from build123d import *

# Parameters (mm, degrees)
EXTRUDE_1_DEPTH        = 25
SKETCH_4_R             = 22
CUT_EXTRUDE_1_DEPTH    = 1.8
CUT_EXTRUDE_START      = 6
CUT_EXTRUDE_1_2_DEPTH  = 3
SKETCH_11_W            = 18.9
SKETCH_11_H            = 1.4
EXTRUDE_3_DEPTH        = 1.5
FILLET_1_R             = 0.25
SKETCH_12_R            = 1
CUT_EXTRUDE_2623_DEPTH = 91.722501261
CUT_EXTRUDE_1_3_DEPTH  = 1
SKETCH_14_W            = 0.8
SKETCH_14_H            = 6.2
CUT_EXTRUDE_2_DEPTH    = 1


with BuildPart() as part:
    # 草图2 → 整体拉伸-薄壁1 (new, symmetric)
    with BuildSketch(Plane.XY):
        with BuildLine():
            ThreePointArc((28.874192719, 5.049687275), (37.065713162, 9.313922912), (38.271118927, 18.469888708))
            Line((38.271118927, 18.469888708), (10.23281379, 95.504498952))
            Line((10.23281379, 95.504498952), (13.051891653, 96.530559382))
            Line((13.051891653, 96.530559382), (41.090196789, 19.495949138))
            ThreePointArc((41.090196789, 19.495949138), (39.523169295, 7.593193603), (28.874192719, 2.049687275))
            Line((28.874192719, 2.049687275), (28.874192719, 5.049687275))
        make_face()
    extrude(amount=EXTRUDE_1_DEPTH, both=True)

    # 草图4 → Cut-Extrude 1 (cut)
    with BuildSketch(Plane(origin=(42.549434126, 15.486727507, 0), x_dir=(0, 0, -1), z_dir=(0.9396926207859071, 0.3420201433256726, 0))):
        with Locations(Location((0, 60.845044478, 0), (0, 0, 90))):
            Circle(SKETCH_4_R)
    extrude(amount=-CUT_EXTRUDE_1_DEPTH, mode=Mode.SUBTRACT)

    # 草图3 → Cut-Extrude 1 2 (cut)
    with BuildSketch(Plane.XY.offset(CUT_EXTRUDE_START)):
        with BuildLine():
            ThreePointArc((28.874192719, 3.849687275), (38.048695615, 8.625631188), (39.398750072, 18.88031288))
            Line((39.398750072, 18.88031288), (27.572199729, 51.373492899))
            Line((27.572199729, 51.373492899), (26.546139299, 54.192570761))
            Line((26.546139299, 54.192570761), (28.237586016, 54.808207019))
            Line((28.237586016, 54.808207019), (29.263646446, 51.989129157))
            Line((29.263646446, 51.989129157), (41.090196789, 19.495949138))
            ThreePointArc((41.090196789, 19.495949138), (39.523169295, 7.593193603), (28.874192719, 2.049687275))
            Line((28.874192719, 2.049687275), (28.874192719, 3.849687275))
        make_face()
    cut_extrude_1_2 = extrude(amount=-CUT_EXTRUDE_1_2_DEPTH, mode=Mode.SUBTRACT)

    # 镜向1: Cut-Extrude 1 2 across plane
    add(cut_extrude_1_2.mirror(Plane.XY), mode=Mode.SUBTRACT)

    # 草图11 → 底部卡扣凸台-拉伸3 (add)
    with BuildSketch(Plane.ZY.offset(-28.874192719)):
        with Locations((-15.55, 2.749687275)):
            Rectangle(SKETCH_11_W, SKETCH_11_H)
        with Locations((15.55, 2.749687275)):
            Rectangle(SKETCH_11_W, SKETCH_11_H)
    extrude(amount=EXTRUDE_3_DEPTH)

    # 底部卡扣圆角1
    fillet_1_edges = [part.edges().sort_by_distance(p)[0] for p in [
        (27.374192719, 2.749687275, -25),
        (27.374192719, 2.049687275, -15.55),
        (27.374192719, 2.749687275, -6.1),
        (27.374192719, 3.449687275, -15.55),
        (27.374192719, 2.749687275, 6.1),
        (27.374192719, 2.049687275, 15.55),
        (27.374192719, 2.749687275, 25),
        (27.374192719, 3.449687275, 15.55),
    ]]
    fillet(fillet_1_edges, radius=FILLET_1_R)

    # 草图12 → Cut-Extrude 2623 (cut, through all)
    with BuildSketch(Plane(origin=(39.730356264, 14.460667077, 0), x_dir=(0, 0, 1), z_dir=(-0.9396926207859071, -0.3420201433256726, 0))):
        with Locations(Location((23, 80.282840932, 0), (0, 0, 270))):
            Circle(SKETCH_12_R)
        with Locations(Location((-23, 80.282840932, 0), (0, 0, 270))):
            Circle(SKETCH_12_R)
    extrude(amount=-CUT_EXTRUDE_2623_DEPTH, mode=Mode.SUBTRACT)

    # 草图13 → Cut-Extrude 1 3 (cut)
    with BuildSketch(Plane(origin=(39.730356264, 14.460667077, 0), x_dir=(0, 0, 1), z_dir=(-0.9396926207859071, -0.3420201433256726, 0))):
        with BuildLine():
            Line((23, 82.282840932), (25, 82.282840932))
            Line((25, 82.282840932), (25, 78.282840932))
            Line((25, 78.282840932), (23, 78.282840932))
            ThreePointArc((23, 78.282840932), (21, 80.282840932), (23, 82.282840932))
        make_face()
        with BuildLine():
            Line((-25, 82.282840932), (-25, 78.282840932))
            Line((-25, 78.282840932), (-23, 78.282840932))
            ThreePointArc((-23, 78.282840932), (-21, 80.282840932), (-23, 82.282840932))
            Line((-23, 82.282840932), (-25, 82.282840932))
        make_face()
    extrude(amount=-CUT_EXTRUDE_1_3_DEPTH, mode=Mode.SUBTRACT)

    # 草图14 → 切除-拉伸2 (cut)
    with BuildSketch(Plane(origin=(-29.497542473, 81.043831875, 0), x_dir=(0.9396926207859067, 0.3420201433256736, 0), z_dir=(-0.3420201433256736, 0.9396926207859068, 0))):
        with Locations((43.680162028, 0)):
            Rectangle(SKETCH_14_W, SKETCH_14_H)
    extrude(amount=-CUT_EXTRUDE_2_DEPTH, mode=Mode.SUBTRACT)


solid = part.part
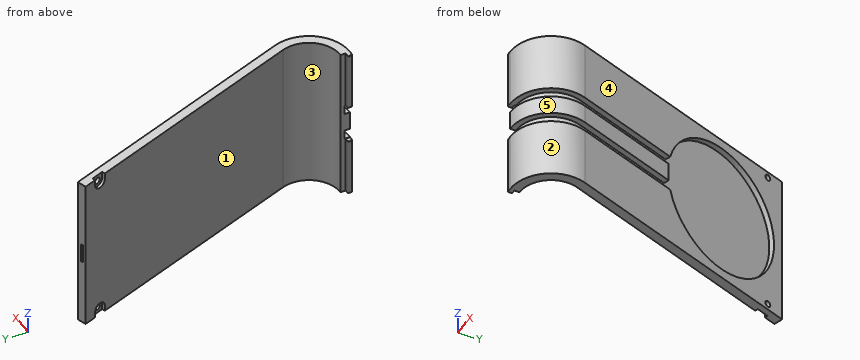
Work out the finished part from the listing and answer in its coordinate system (mm). Face numbers are marked on the shaded views. A direction names the side the tool comes from. Give positions to 0.01 mm unless a question says otherwise; leave off trailing zeros. Loops run counter-clockwise (first coordinate to the right, second up) from the corner with the lowest first, then second, coordinate; pieces in that order, holes last. Notation, with made-up numbers: (87.5, -38) - (129.5, -38) arc R19 ccw to (129.5, -21) - close; hole circle Ø10 at (-25.5, 58). An arc over 180 degrees is marked (long way). Answer in a Markdown table with one row per item. Add a question column.
Q1. A tool of negligible diameter and unlimited length cuts with its end or side. For the marked faces 1 and 2, from which of +Z, -Z, +X, -X, +Y, -Y can it reach the whole face along a straight path? Write none if from no direction.
Q2. Each of these flat-tipped pins is pushed along its axis until it touches: P1, Ø1, axis at y = 2.5, z = -16, coming from the -X side; P2, Ø10, axis at y = 26.5, z = -16.5, coming from the +X side; P3, Ø2, axis at y = 49.5, z = -8.5, coming from the -X side. Where does it stop, or does it pass through?
Q3. The part is cut by section D-D (z = -18.5). Determine the outline of the cut face in (x, y).
Q4. The part is cut by section A-A (x = 34.5). Determine the outline of the cut face in (y, z).
Q5. Consider line 1 along X through (y, z) = (35, 4); line 2 along X through (y, z) = (52.5, 1). Determine where each line is inside the solid, lowest interval first.
Q6. The part is cut by section B-B (z = 12). Determine the outline of the cut face in (x, y), and give its area (3 significant figures).
Q7. The part is cut by section C-C (y = 8.5). Determine the outline of the cut face in (x, z), and give its area (3 significant figures).
Q8. Determine the mould class of the marked faces 3, 4 and 5 for opening direction Y: released by +Y, released by -Y, zero draft, split by the parting line, or undercut.
Solution:
| question | item | result |
|---|---|---|
| 1 | face 1 | +Z, -Z, -X |
| 1 | face 2 | +Z, -Z, +X |
| 2 | P1 | stops at x = 27.37 |
| 2 | P2 | stops at x = 40.36 |
| 2 | P3 | stops at x = 26.61 |
| 3 | outline | (10.23, 95.5) - (38.27, 18.47) arc R10 cw to (28.87, 5.05) - (28.87, 3.45) - (27.62, 3.45) arc R0.25 ccw to (27.37, 3.2) - (27.37, 2.3) arc R0.25 ccw to (27.62, 2.05) - (28.87, 2.05) arc R13 ccw to (41.09, 19.5) - (25.81, 61.47) - (24.12, 60.86) - (15.98, 83.23) - (17.67, 83.85) - (13.05, 96.53) - close |
| 4 | outline | (3.33, -25) - (6.78, -25) - (6.78, 25) - (3.33, 25) - (3.33, 6) - (5.37, 6) - (5.37, 3) - (3.33, 3) - (3.33, -3) - (5.37, -3) - (5.37, -6) - (3.33, -6) - close; (28.83, -25) - (37.6, -25) - (37.6, -6) - (32.34, -6) - (32.34, -3) - (37.6, -3) - (37.6, 3) - (32.34, 3) - (32.34, 6) - (37.6, 6) - (37.6, 25) - (28.83, 25) - close |
| 5 | line 1 | x = 32.25 to 33.53 |
| 5 | line 2 | x = 25.89 to 27.16 |
| 6 | outline | (10.23, 95.5) - (38.27, 18.47) arc R10 cw to (28.87, 5.05) - (28.87, 3.45) - (27.62, 3.45) arc R0.25 ccw to (27.37, 3.2) - (27.37, 2.3) arc R0.25 ccw to (27.62, 2.05) - (28.87, 2.05) arc R13 ccw to (41.09, 19.5) - (28.05, 55.34) - (26.35, 54.72) - (13.74, 89.37) - (15.43, 89.99) - (13.05, 96.53) - close |
| 6 | area | 248 mm² |
| 7 | outline | (36.43, -25) - (40.1, -25) - (40.1, -6) - (37.96, -6) - (37.96, -3) - (40.1, -3) - (40.1, 3) - (37.96, 3) - (37.96, 6) - (40.1, 6) - (40.1, 25) - (36.43, 25) - close |
| 7 | area | 171 mm² |
| 8 | face 3 | undercut |
| 8 | face 4 | released by +Y |
| 8 | face 5 | split by the parting line |
